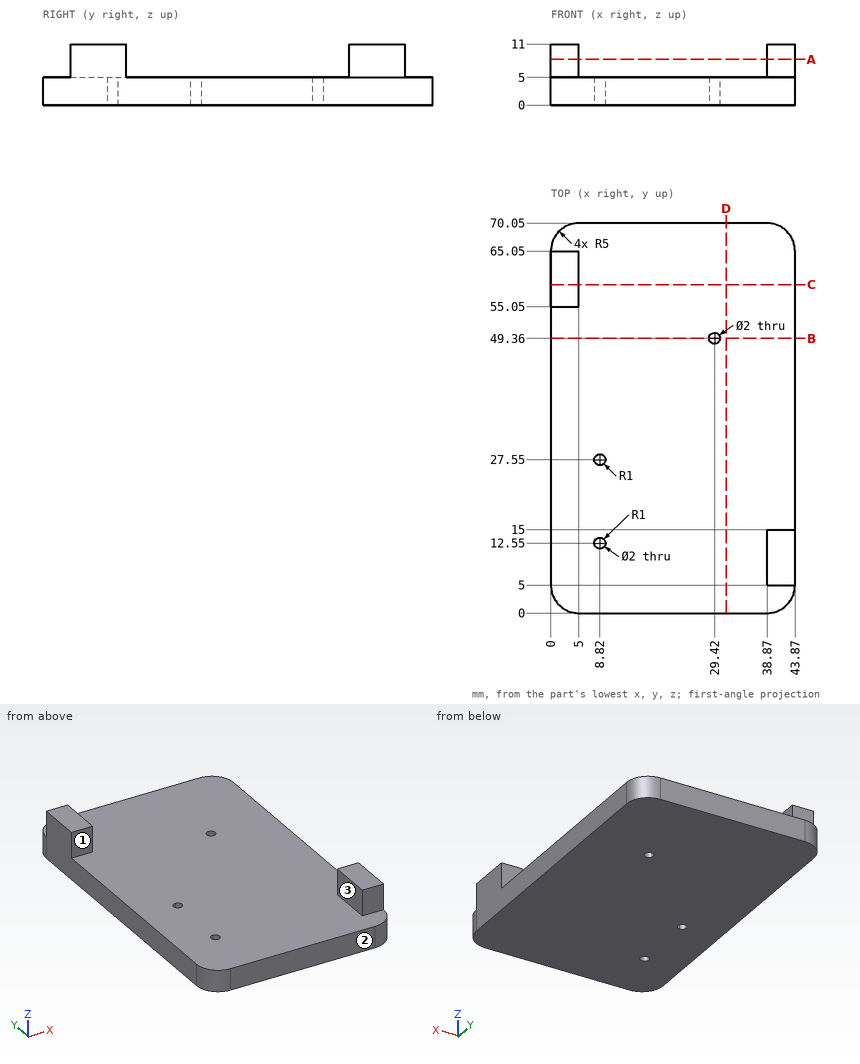
Check sheet for the drawn part. Datum: minimum x, y, z corner. Units: mm. A direction names the side the tool comes from. Give positions to 0.01 mm unless a question says otherwise; leave off trailing zeros. Write each loop counter-clockwise with the first axis right and the second up, starting at its lowest first coordinate (ties: lowest second). Pieces come first, ordered by that corner, then holes.
(1) Cross-section at A-A (z = 8.25). Enter the section's corners in (x, y).
(2) Cross-section at D-D (x = 31.5). Enter the section's corners in (y, z).
(3) Cross-section at B-B (y = 49.36). Enter the section's corners in (x, z).
(4) Access from +Z, -Z, +X, -X, +Y, -Y to the whole of each face (thin tool, end or side, straight path). Record for the marked faces 1, 2 and 3.
(5) Gauge pin test, flat ends, axial feed: pin 1 (22 mm diameter, centred on x = 18.5, y = 22.5, fed in from +Z); pin 2 (6.5 mm diameter, centred on y = 12.5, z = 8, fed in from -X); pin 3 (5.5 mm diameter, centred on x = 41.5, z = 7.5, fed in from +Y); pin 4 (1.5 mm diameter, centred on x = 40.5, z = 9, fed in from -Y). Record the tip position at first contact, or that the pin passes through.
(6) Material ranges on line 1 (Y direction, x = 8.82, z = 2.5); line 2 (Y direction, x = 29.42, z = 1.25); line 3 (X direction, y = 12.55, z = 3.3), recorded low to high.
(7) Cross-section at C-C (y = 59). Enter the section's corners in (x, z), plus the area to 3 significant figures.
Worked out:
1. outline: (0, 55.05) - (5, 55.05) - (5, 65.05) - (0, 65.05) - close; (38.87, 5) - (43.87, 5) - (43.87, 15) - (38.87, 15) - close
2. outline: (0, 0) - (70.05, 0) - (70.05, 5) - (0, 5) - close
3. outline: (0, 0) - (28.42, 0) - (28.42, 5) - (0, 5) - close; (30.42, 0) - (43.87, 0) - (43.87, 5) - (30.42, 5) - close
4. face 1: +Z, +X, -X, -Y
4. face 2: +Z, -Z, +X, -X, -Y
4. face 3: +Z, -X, +Y, -Y
5. pin 1: stops at z = 5
5. pin 2: stops at x = 0
5. pin 3: stops at y = 69.82
5. pin 4: stops at y = 5
6. line 1: y = 0 to 11.55, 13.55 to 26.55, 28.55 to 70.05
6. line 2: y = 0 to 48.36, 50.36 to 70.05
6. line 3: x = 0 to 7.82, 9.82 to 43.87
7. outline: (0, 0) - (43.87, 0) - (43.87, 5) - (5, 5) - (5, 11) - (0, 11) - close
7. area: 249 mm2
